```python
from build123d import *

# Parameters (mm, degrees)
SKETCH1_R           = 75
SKETCH1_R_2         = 11
BOSS_EXTRUDE1_DEPTH = 12
SKETCH2_R           = 2.75
CUT_EXTRUDE1_DEPTH  = 107.742681248
SKETCH3_R           = 5.25
CUT_EXTRUDE2_DEPTH  = 6
SKETCH4_R           = 62.1
CUT_EXTRUDE3_DEPTH  = 2
SKETCH5_R           = 2.75
CUT_EXTRUDE4_DEPTH  = 107.742681248
SKETCH8_R           = 5.5
CUT_EXTRUDE5_DEPTH  = 5
FILLET1_R           = 0.5
CHAMFER1_SIZE       = 1
CHAMFER2_SIZE       = 1
CHAMFER3_SIZE       = 1
CHAMFER4_SIZE       = 0.5


with BuildPart() as part:
    # Sketch1 → Boss-Extrude1 (new body)
    with BuildSketch(Plane(origin=(0, 0, 0), x_dir=(1, 0, 0), z_dir=(0, 1, 0))):
        with Locations(Location((0, 0, 0), (0, 0, 270))):
            Circle(SKETCH1_R)
        with Locations(Location((0, 0, 0), (0, 0, 270))):
            Circle(SKETCH1_R_2, mode=Mode.SUBTRACT)
    extrude(amount=BOSS_EXTRUDE1_DEPTH)

    # Sketch2 → Cut-Extrude1 (cut, through all)
    with BuildSketch(Plane(origin=(0, 12, 0), x_dir=(1, 0, 0), z_dir=(0, 1, 0))):
        with Locations(Location((-23.57, 23.57, 0), (0, 0, 270))):
            Circle(SKETCH2_R)
        with Locations(Location((23.57, 23.57, 0), (0, 0, 270))):
            Circle(SKETCH2_R)
        with Locations(Location((-23.57, -23.57, 0), (0, 0, 270))):
            Circle(SKETCH2_R)
        with Locations(Location((23.57, -23.57, 0), (0, 0, 270))):
            Circle(SKETCH2_R)
    extrude(amount=-CUT_EXTRUDE1_DEPTH, mode=Mode.SUBTRACT)

    # Sketch3 → Cut-Extrude2 (cut)
    with BuildSketch(Plane(origin=(0, 12, 0), x_dir=(1, 0, 0), z_dir=(0, 1, 0))):
        with Locations(Location((-23.57, 23.57, 0), (0, 0, 270))):
            Circle(SKETCH3_R)
        with Locations(Location((23.57, 23.57, 0), (0, 0, 270))):
            Circle(SKETCH3_R)
        with Locations(Location((-23.57, -23.57, 0), (0, 0, 270))):
            Circle(SKETCH3_R)
        with Locations(Location((23.57, -23.57, 0), (0, 0, 270))):
            Circle(SKETCH3_R)
    extrude(amount=-CUT_EXTRUDE2_DEPTH, mode=Mode.SUBTRACT)

    # Sketch4 → Cut-Extrude3 (cut)
    with BuildSketch(Plane(origin=(0, 12, 0), x_dir=(1, 0, 0), z_dir=(0, 1, 0))):
        with Locations(Location((0, 0, 0), (0, 0, 270))):
            Circle(SKETCH4_R)
    extrude(amount=-CUT_EXTRUDE3_DEPTH, mode=Mode.SUBTRACT)

    # Sketch5 → Cut-Extrude4 (cut, through all)
    with BuildSketch(Plane(origin=(0, 12, 0), x_dir=(1, 0, 0), z_dir=(0, 1, 0))):
        with Locations(Location((0, 68, 0), (0, 0, 270))):
            Circle(SKETCH5_R)
        with Locations(Location((48.083261121, 48.083261121, 0), (0, 0, 270))):
            Circle(SKETCH5_R)
        with Locations(Location((68, 0, 0), (0, 0, 270))):
            Circle(SKETCH5_R)
        with Locations(Location((48.083261121, -48.083261121, 0), (0, 0, 270))):
            Circle(SKETCH5_R)
        with Locations(Location((0, -68, 0), (0, 0, 270))):
            Circle(SKETCH5_R)
        with Locations(Location((-48.083261121, -48.083261121, 0), (0, 0, 270))):
            Circle(SKETCH5_R)
        with Locations(Location((-68, 0, 0), (0, 0, 270))):
            Circle(SKETCH5_R)
        with Locations(Location((-48.083261121, 48.083261121, 0), (0, 0, 270))):
            Circle(SKETCH5_R)
        with Locations(Location((26.022473401, 62.823808211, 0), (0, 0, 270))):
            Circle(SKETCH5_R)
        with Locations(Location((62.823808211, -26.022473401, 0), (0, 0, 270))):
            Circle(SKETCH5_R)
        with Locations(Location((-26.022473401, -62.823808211, 0), (0, 0, 270))):
            Circle(SKETCH5_R)
        with Locations(Location((-62.823808211, 26.022473401, 0), (0, 0, 270))):
            Circle(SKETCH5_R)
    extrude(amount=-CUT_EXTRUDE4_DEPTH, mode=Mode.SUBTRACT)

    # Sketch8 → Cut-Extrude5 (cut)
    with BuildSketch(Plane.XZ):
        with Locations(Location((0, 68, 0), (0, 0, 270))):
            Circle(SKETCH8_R)
        with Locations(Location((-48.083261121, 48.083261121, 0), (0, 0, 270))):
            Circle(SKETCH8_R)
        with Locations(Location((48.083261121, 48.083261121, 0), (0, 0, 270))):
            Circle(SKETCH8_R)
        with Locations(Location((48.083261121, -48.083261121, 0), (0, 0, 270))):
            Circle(SKETCH8_R)
        with Locations(Location((0, -68, 0), (0, 0, 270))):
            Circle(SKETCH8_R)
        with Locations(Location((-48.083261121, -48.083261121, 0), (0, 0, 270))):
            Circle(SKETCH8_R)
        with Locations(Location((-68, 0, 0), (0, 0, 270))):
            Circle(SKETCH8_R)
        with Locations(Location((68, 0, 0), (0, 0, 270))):
            Circle(SKETCH8_R)
    extrude(amount=-CUT_EXTRUDE5_DEPTH, mode=Mode.SUBTRACT)

    # Fillet1
    fillet1_edges = [part.edges().sort_by_distance(p)[0] for p in [
        (0, 10, -62.1),
    ]]
    fillet(fillet1_edges, radius=FILLET1_R)

    # Chamfer1
    chamfer1_edges = [part.edges().sort_by_distance(p)[0] for p in [
        (0, 12, -62.1),
    ]]
    chamfer(chamfer1_edges, length=CHAMFER1_SIZE)

    # Chamfer2
    chamfer2_edges = [part.edges().sort_by_distance(p)[0] for p in [
        (-48.083261121, 12, -50.833261121),
        (62.823808211, 12, 23.272473401),
        (-26.022473401, 12, 60.073808211),
        (-62.823808211, 12, -28.772473401),
        (0, 12, -70.75),
        (23.57, 10, -28.82),
        (-23.57, 10, 18.32),
        (23.57, 10, 18.32),
        (-23.57, 10, -28.82),
        (26.022473401, 12, -65.573808211),
        (48.083261121, 12, -50.833261121),
        (68, 12, -2.75),
        (48.083261121, 12, 45.333261121),
        (0, 12, 65.25),
        (-48.083261121, 12, 45.333261121),
        (-68, 12, -2.75),
    ]]
    chamfer(chamfer2_edges, length=CHAMFER2_SIZE)

    # Chamfer3
    chamfer3_edges = [part.edges().sort_by_distance(p)[0] for p in [
        (0, 0, 73.5),
        (68, 0, 5.5),
        (-68, 0, 5.5),
        (-48.083261121, 0, -42.583261121),
        (0, 0, -62.5),
        (48.083261121, 0, -42.583261121),
        (48.083261121, 0, 53.583261121),
        (-48.083261121, 0, 53.583261121),
    ]]
    chamfer(chamfer3_edges, length=CHAMFER3_SIZE)

    # Chamfer4
    chamfer4_edges = [part.edges().sort_by_distance(p)[0] for p in [
        (23.57, 6, -26.32),
        (-23.57, 6, 20.82),
        (23.57, 6, 20.82),
        (-23.57, 6, -26.32),
    ]]
    chamfer(chamfer4_edges, length=CHAMFER4_SIZE)


solid = part.part
```
Here's how the part is built. I have some questions about the finished solid (model axes, mm). A direction names the side the tool comes from. Give positions to 0.01 mm unless a question says otherwise; leave off trailing zeros. Use one line per item in the form item = value.
1) Suppose I cut it at A-A (x = 0). Give the number of separate pieces and of enclosed holes in the cut face, and give its area (3 significant figures).
Verdict:
separate_pieces = 4
enclosed_holes = 0
area = 1,140 mm2
2) On a 3-axis mill with a long thin cutter (end or side, diameter ignored), from which of +Z, -Z, +X, -X, +Y, -Y can I reach the whole of each face in a straight line? I mean faces 1 (the face through (3, 5, 67)), 2 (the face through (28.775, 7.521, -24.253)), 3 (the face through (64.682, 5.577, 23.996)). Say none if no direction works.
Verdict:
face_1 = -Y
face_2 = +Y
face_3 = +Y, -Y
3) If I drill on L1, parallel to X at y = 3, z = 0; L2, parallel to Z at x = -28, y = 7.25; L3, parallel to Z at x = -19.5, y = 6.5, over which ranges is the centre line in solid material (lowest first)? Write a range as [from, to].
Verdict:
L1 = [-75, -73.5], [-62.5, -11], [11, 62.5], [73.5, 75]
L2 = [-69.58, -26.39], [-20.75, 20.75], [26.39, 60.91], [64.73, 69.58]
L3 = [-72.42, -26.89], [-20.25, 20.25], [26.89, 72.42]
4) I'm going to push flat-ended pins straight in: pin 1 (6.5 mm diameter, centred on x = 0, z = -68, fed in from +Y); pin 2 (2 mm diameter, centred on x = 55.5, y = 7, fed in from -Z); pin 3 (4 mm diameter, centred on x = 9.5, z = 33.5, fed in from +Y). Where does each tip first touch, or does it pass through?
Verdict:
pin_1 = 11.5
pin_2 = -51.52
pin_3 = 10
